from build123d import *

# Parameters (mm, degrees)
BASE_FLANGE1_DEPTH        = 44.45
EDGE_FLANGE1_DEPTH        = 43.7134
EDGE_FLANGE1_START        = 1.5875
EDGE_FLANGE1_FLAT_DEPTH   = 1.5875
EDGE_FLANGE1_BEND_DEPTH   = 43.7134
EDGE_FLANGE1_FLAT_2_DEPTH = 1.5875
SKETCH12_R                = 14.2875
CUT_EXTRUDE1_DEPTH        = 88.025228164
SKETCH13_R                = 3.3782
CUT_EXTRUDE2_DEPTH        = 88.025228164


# Sheet-metal steps are written as plain solids
with BuildPart() as part:
    # Sketch1 → Base-Flange1 (new body)
    with BuildSketch(Plane(origin=(0, 0, 0), x_dir=(0, 0, -1), z_dir=(1, 0, 0))):
        with BuildLine():
            Line((0, 0), (43.7134, 0))
            ThreePointArc((43.7134, 0), (44.234254855, 0.215745145), (44.45, 0.7366))
            Line((44.45, 0.7366), (44.45, 57.15))
            Line((44.45, 57.15), (46.0375, 57.15))
            Line((46.0375, 57.15), (46.0375, 0.7366))
            ThreePointArc((46.0375, 0.7366), (45.35678687, -0.90678687), (43.7134, -1.5875))
            Line((43.7134, -1.5875), (0, -1.5875))
            Line((0, -1.5875), (0, 0))
        make_face()
    extrude(amount=BASE_FLANGE1_DEPTH)

    # Edge-Flange1 bend section (across the edge) → Edge-Flange1 (add)
    with BuildSketch(Plane(origin=(-0.7366, 0, -43.7134), x_dir=(1, 0, 0), z_dir=(0, 0, 1))):
        with BuildLine():
            Line((-1.5875, 0.7366), (0, 0.7366))
            ThreePointArc((0, 0.7366), (0.215745145, 0.215745145), (0.7366, 0))
            Line((0.7366, 0), (0.7366, -1.5875))
            ThreePointArc((0.7366, -1.5875), (-0.90678687, -0.90678687), (-1.5875, 0.7366))
        make_face()
    extrude(amount=EDGE_FLANGE1_DEPTH)

    # Edge-Flange1 profile (on flange) → Edge-Flange1 flat (add)
    with BuildSketch(Plane.ZY.offset(0.7366).offset(EDGE_FLANGE1_START)):
        Polygon((0, 0.7366), (0, 6.35), (-37.3634, 57.15), (-43.7134, 57.15), (-43.7134, 0.7366), align=None)
    extrude(amount=-EDGE_FLANGE1_FLAT_DEPTH)

    # Edge-Flange1 bend section 2 (across the edge) → Edge-Flange1 bend (add)
    with BuildSketch(Plane(origin=(45.1866, 0, 0), x_dir=(-1, 0, 0), z_dir=(0, 0, -1))):
        with BuildLine():
            Line((-1.5875, 0.7366), (0, 0.7366))
            ThreePointArc((0, 0.7366), (0.215745145, 0.215745145), (0.7366, 0))
            Line((0.7366, 0), (0.7366, -1.5875))
            ThreePointArc((0.7366, -1.5875), (-0.90678687, -0.90678687), (-1.5875, 0.7366))
        make_face()
    extrude(amount=EDGE_FLANGE1_BEND_DEPTH)

    # Edge-Flange1 profile 2 (on flange) → Edge-Flange1 flat 2 (add)
    with BuildSketch(Plane(origin=(45.1866, 0, 0), x_dir=(0, 0, -1), z_dir=(1, 0, 0)).offset(EDGE_FLANGE1_START)):
        Polygon((0, 6.35), (0, 0.7366), (43.7134, 0.7366), (43.7134, 57.15), (37.3634, 57.15), align=None)
    extrude(amount=-EDGE_FLANGE1_FLAT_2_DEPTH)

    # Sketch12 → Cut-Extrude1 (cut, through all)
    with BuildSketch(Plane(origin=(0, 0, -46.0375), x_dir=(-1, 0, 0), z_dir=(0, 0, -1))):
        with Locations((-22.225, 34.925)):
            Circle(SKETCH12_R)
    extrude(amount=-CUT_EXTRUDE1_DEPTH, mode=Mode.SUBTRACT)

    # Sketch13 → Cut-Extrude2 (cut, through all)
    with BuildSketch(Plane(origin=(0, 0, 0), x_dir=(1, 0, 0), z_dir=(0, 1, 0))):
        with Locations(Location((38.0844298, 11.2395, 0), (0, 0, 270))):
            Circle(SKETCH13_R)
        with Locations(Location((6.3344298, 20.235970884, 0), (0, 0, 270))):
            Circle(SKETCH13_R)
    extrude(amount=-CUT_EXTRUDE2_DEPTH, mode=Mode.SUBTRACT)


solid = part.part
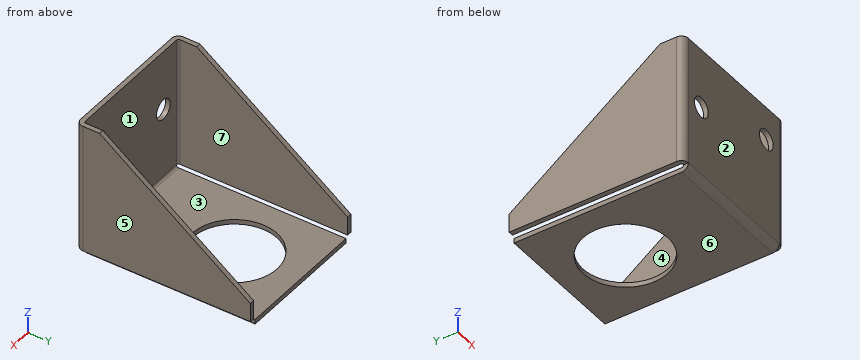
Source: CAD feature listing. Evaluate the final solid. Frame: model axes, mm. Face numbers are marked on the shaded views. A direction names the side the tool comes from. Give positions to 0.01 mm unless a question says otherwise; leave off trailing zeros. Write each loop counter-clockwise with the first axis right and the second up, starting at its lowest first coordinate (ties: lowest second). Pieces come first, ordered by that corner, then holes. Notation, with made-up numbers: M -4,11 L 14,11 A33 ccw 14,50 Z; hole C -2.75,30 d3. An arc over 180 degrees is marked long. Return JSON: item names as keys, results as strings. Group by question number.
1) Draft query along X for the marked faces 4, 5, 6 and 7. Return one class per face: released by +X, released by -X, zero draft, split by the parting line, or undercut.
2) Set-up query: the marked faces 1, 2 and 3. Return all of +Z, -Z, +X, -X, +Y, -Y with unobstructed straight access to the full face (end or side cutting, diameter ignored); none if empty.
3) Ray query, L1, parallel to X at y = 20, z = -22; L2, parallel to Z at x = 29.5, y = 17; L3, parallel to Y at x = 23, z = -39.5. Return the intervals inside material, ascending.
4) First-contact query: pin 1 Ø0.7 at (x, y) = (-0.5, 28.5) entering from -Z; pin 2 Ø4 at (x, y) = (34, 49) entering from +Z; pin 3 Ø1.2 at (y, z) = (33.5, -44.5) entering from +X; pin 4 Ø6 at (x, z) = (6.33, -20.24) entering from +Y. Flat tips, straight axial feed; report the tip coordinate or a pass-through.
5) Cut plane C-C, the plane z = -10. Output: boundary loops of the cut face in (x, y).
6) Cut plane D-D, the plane z = -38.5. Output: boundary loops of the cut face in (x, y).
7) Cut plane B-B, the plane x = 35.5. Output: boundary loops of the cut face in (y, z).
8) Cut plane A-A, the plane y = 3.5. Output: boundary loops of the cut face in (x, z), then the cut area to 3 significant figures.
Data:
{
 "1": {"face 4": "undercut", "face 5": "released by +X", "face 6": "zero draft", "face 7": "undercut"},
 "2": {"face 1": "+Z, +Y", "face 2": "+Z, -Z, +X, -X, -Y", "face 3": "+Z, +X, -X, +Y"},
 "3": {"L1": "x = -2.32 to -0.74, 45.19 to 46.77", "L2": "z = -46.04 to -44.45", "L3": "y = -1.59 to 0"},
 "4": {"pin 1": "stops at z = -43.71", "pin 2": "stops at z = -44.45", "pin 3": "stops at x = 44.45", "pin 4": "passes through"},
 "5": {"outline": "M -2.32,0.74 A2.32 ccw 0,-1.59 L 34.94,-1.59 L 34.94,0 L 0,0 A0.74 cw -0.74,0.74 L -0.74,19.95 L -2.32,19.95 Z; M 41.23,-1.59 L 44.45,-1.59 A2.32 ccw 46.77,0.74 L 46.77,19.95 L 45.19,19.95 L 45.19,0.74 A0.74 cw 44.45,0 L 41.23,0 Z"},
 "6": {"outline": "M -2.32,0.74 A2.32 ccw 0,-1.59 L 44.45,-1.59 A2.32 ccw 46.77,0.74 L 46.77,57.15 L 45.19,57.15 L 45.19,0.74 A0.74 cw 44.45,0 L 0,0 A0.74 cw -0.74,0.74 L -0.74,57.15 L -2.32,57.15 Z"},
 "7": {"outline": "M -1.59,-43.71 A2.32 ccw 0.74,-46.04 L 29.64,-46.04 L 29.64,-44.45 L 0.74,-44.45 A0.74 cw 0,-43.71 L 0,-13.42 L -1.59,-13.42 Z; M -1.59,-9.06 L 0,-9.06 L 0,0 L -1.59,0 Z; M 40.21,-46.04 L 57.15,-46.04 L 57.15,-44.45 L 40.21,-44.45 Z"},
 "8": {"outline": "M -2.32,-43.71 L -0.74,-43.71 L -0.74,0 L -2.32,0 Z; M 0,-46.04 L 44.45,-46.04 L 44.45,-44.45 L 0,-44.45 Z; M 45.19,-43.71 L 46.77,-43.71 L 46.77,0 L 45.19,0 Z", "area": "209 mm²"}
}
